Geometry check sheet. Reference: drawing and pictorial views, mm from the part's lowest x, y, z. Round coordinates to 2 decimals unless told otherwise and drop trailing zeros. Order: outer loops, then holes, each group sorted by start corner. A loop starts at its lowest first (then second) coordinate and runs counter-clockwise, first axis right, second up.
(1) Sectioned sample at A-A, the plane y = 7.5. Enter the section's corners in (x, z).
(2) Sectioned sample at C-C, the plane y = 4. Enter the section's corners in (x, z).
(3) Sectioned sample at B-B, the plane z = 1.9. Enter the section's corners in (x, y).
(4) Thickness scan on probe 1 along Y at (x, z) = (1.55, 1.9); probe 2 along X at (y, z) = (5.25, 1); probe 3 along Y at (x, z) = (0.5, 1.75). Record the ranges inside material, lowest first.
(5) Mould release check, pull along Z, two halves, no side actions. Record for the marked faces 1, 2 and 3: released by +Z, released by -Z, zero draft, split by the parting line, or undercut.
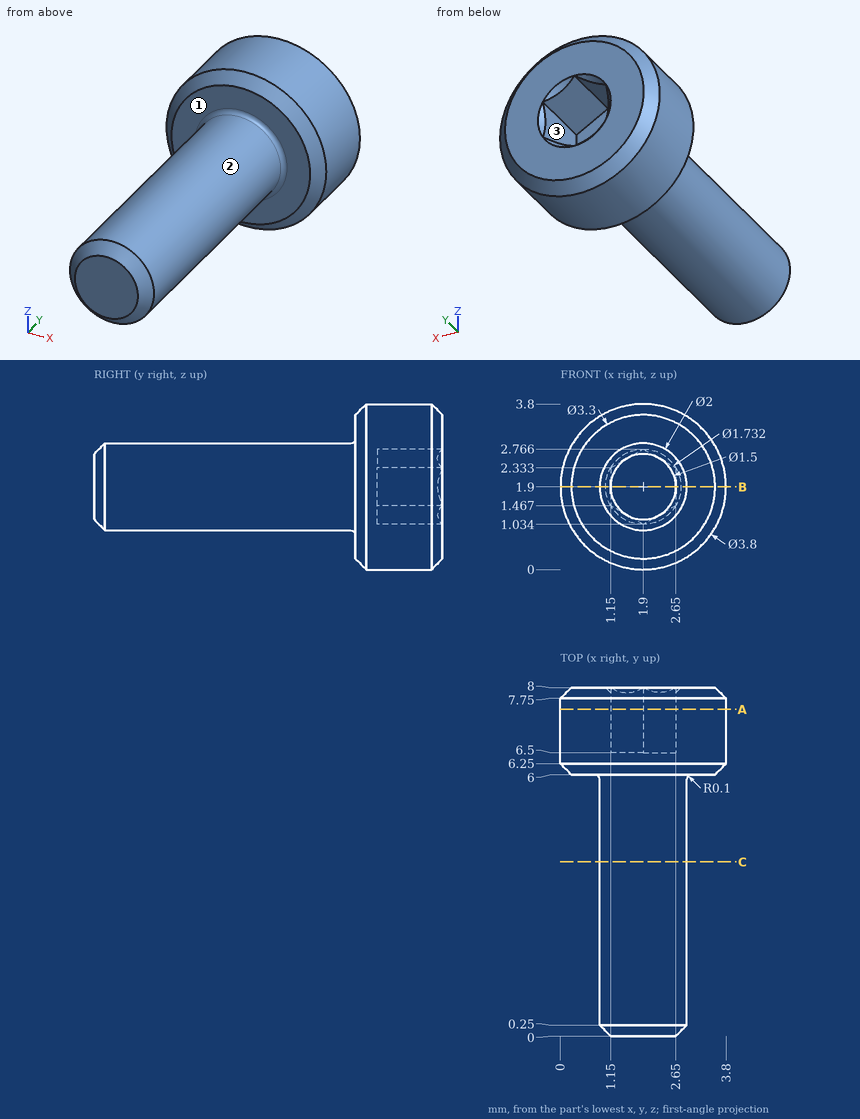
Derived:
1. outline: circle Ø3.8 at (1.9, 1.9); hole (1.15, 1.47) - (1.9, 1.03) - (2.65, 1.47) - (2.65, 2.33) - (1.9, 2.77) - (1.15, 2.33) - close
2. outline: circle Ø2 at (1.9, 1.9)
3. outline: (0, 6.25) - (0.25, 6) - (0.8, 6) arc R0.1 cw to (0.9, 5.9) - (0.9, 0.25) - (1.15, 0) - (2.65, 0) - (2.9, 0.25) - (2.9, 5.9) arc R0.1 cw to (3, 6) - (3.55, 6) - (3.8, 6.25) - (3.8, 7.75) - (3.55, 8) - (2.77, 8) - (2.65, 7.88) - (2.65, 6.5) - (1.15, 6.5) - (1.15, 7.88) - (1.03, 8) - (0.25, 8) - (0, 7.75) - close
4. probe 1: y = 0 to 6.5
4. probe 2: x = 1.46 to 2.34
4. probe 3: y = 6 to 8
5. face 1: zero draft
5. face 2: split by the parting line
5. face 3: undercut
